```python
from build123d import *

# Parameters (mm, degrees)
F0_R      = 10
F2_R      = 10
F3_FACE_R = 10
F5_R      = 10
F7_R      = 8
F8_DEPTH  = 130.001
F10_DEPTH = 10.001


with BuildPart() as f3:
    # F0 (on Top) → F3 section 0
    with BuildSketch(Plane.XY):
        Circle(F0_R)
    # F2 (on offset) → F3 section 1
    with BuildSketch(Plane.XY.offset(60)):
        Circle(F2_R)
    loft()

    # F3_face (on face) → F6 section 0
    with BuildSketch(Plane(origin=(0, 0, 0), x_dir=(1, 0, 0), z_dir=(0, 0, -1))):
        Circle(F3_FACE_R)
    # F5 (on offset) → F6 section 1
    with BuildSketch(Plane.XY.offset(130)):
        Circle(F5_R)
    loft()

    # F7 (on face) → F8 (cut, through all)
    with BuildSketch(Plane.XY.offset(130)):
        Circle(F7_R)
    extrude(amount=-F8_DEPTH, mode=Mode.SUBTRACT)

    # F9 (on Right) → F10 (cut, through all)
    with BuildSketch(Plane.YZ):
        with BuildLine():
            ThreePointArc((0, 28.75), (0.883883, 29.116117), (1.25, 30))
            ThreePointArc((1.25, 30), (-0.883883, 30.883883), (0, 28.75))
        make_face()
    extrude(amount=-F10_DEPTH, mode=Mode.SUBTRACT)


solid = f3.part
```
Build history of the part. All positions in model axes, mm. Round coordinates to 2 decimals unless told otherwise and drop trailing zeros. Write each loop counter-clockwise with the first axis right and the second up, starting at its lowest first coordinate (ties: lowest second). Pieces come first, ordered by that corner, then holes.
1) Band-saw the part on B-B, the plane y = 4.75. List the corners of the cut face in (x, z).
2) Mould opens along Y. For faces 1 (the flat face through (0, 8.2, 130)), 2 (the cylindrical face through (-1.73, -7.81, 65.91)) say: +Y half, -Y half, draft (parallel to the pull), parting line (faces both ways), or undercut.
3) Band-saw the part on A-A, the plane x = 0. List the corners of the cut face in (y, z), and give its area (3 significant figures).
4) Drill centre lines: probe 1 along Y at (x, z) = (0, 83.5); probe 2 along X at (y, z) = (2.5, 48); probe 3 along X at (y, z) = (7, 105.5). Where is each one in solid material? Low to high.
5) Band-saw the part on C-C, the plane z = 62. List the corners of the cut face in (x, y).
6) Pin check, flat tips, straight feed: pin 1 (5 mm diameter, centred on x = 6.5, z = 63, fed in from +Y); pin 2 (1 mm diameter, centred on y = 6, z = 114, fed in from +X); pin 3 (1 mm diameter, centred on y = -6, z = 61.5, fed in from -X); pin 4 (3 mm diameter, centred on x = -5, y = 0.5, fed in from +Z). Stop position of each tip, or through.
Ans:
1. outline: (-8.8, 0) - (-6.44, 0) - (-6.44, 130) - (-8.8, 130) - close; (6.44, 0) - (8.8, 0) - (8.8, 130) - (6.44, 130) - close
2. face 1: draft
2. face 2: undercut
3. outline: (-10, 0) - (-8, 0) - (-8, 130) - (-10, 130) - close; (8, 0) - (10, 0) - (10, 130) - (8, 130) - close
3. area: 520 mm2
4. probe 1: y = -10 to -8, 8 to 10
4. probe 2: x = -9.68 to -7.6, 7.6 to 9.68
4. probe 3: x = -7.14 to -3.87, 3.87 to 7.14
5. outline: circle Ø20 at (0, 0); hole circle Ø16 at (0, 0)
6. pin 1: stops at y = 9.17
6. pin 2: stops at x = 8.35
6. pin 3: stops at x = -8.35
6. pin 4: passes through
